Autodesk Inventor part; units mm, degrees
ref_plane "作業平面2" through (-125.5285, -9.35, -169.7679) normal (-0.3826834, 0, 0.9238795) x (0.9238795, 0, 0.3826834)
ref_plane "作業平面4" through (-114.2638, -8.3771, -110.4647) normal (0, 0, 1) x (1, 0, 0)
ref_plane "YZ Plane" through (0, 0, 0) normal (1, 0, 0) x (0, 1, 0)
ref_plane "作業平面1" through (-58.5419, 13.75, 0) normal (0, 0, -1) x (-1, 0, 0)
sketch "スケッチ1" plane through (-58.5419, 13.75, 0) normal (0, 0, -1) x (-1, 0, 0)
  line L0 (-47.5988, 17.4243) -> (46.6818, -19.75)
  line L1 (46.6818, -19.75) -> (47.5988, -17.4243)
  line L2 (47.5988, -17.4243) -> (-46.6818, 19.75)
  line L3 (-46.6818, 19.75) -> (-47.5988, 17.4243)
  point P0 (-58.5419, -13.75)
ref_plane "作業平面2" through (-125.5285, -9.35, -169.7679) normal (-0.3826834, 0, 0.9238795) x (0.9238795, 0, 0.3826834)
extrude "押し出し1" add sketch "スケッチ1" along normal up to surface surface through (-125.5285, -9.35, -169.7679) normal (-0.3826834, 0, 0.9238795)
sketch "スケッチ2" plane through (-106.1408, -3.6743, 0) normal (-0.3668097, 0.930296, 0) x (0.930296, 0.3668097, 0)
  circle A0 centre (76.1355, 115.4647) radius 1.5
  circle A1 centre (45.616, 115.4647) radius 1.5
  line L0 (30.3562, 120.4647) -> (30.3562, 110.4647)
  line L1 (91.3953, 120.4647) -> (30.3562, 120.4647)
  line L2 (91.3953, 110.4647) -> (91.3953, 120.4647)
  line L3 (30.3562, 110.4647) -> (91.3953, 110.4647)
  circle A2 centre (76.1355, 5) radius 1.5
  circle A3 centre (45.616, 5) radius 1.5
  line L4 (30.3562, 10) -> (30.3562, 0)
  line L5 (91.3953, 10) -> (30.3562, 10)
  line L6 (91.3953, 0) -> (91.3953, 10)
  line L7 (30.3562, 0) -> (91.3953, 0)
  point P0 (100.0901, 0)
extrude "押し出し2" cut sketch "スケッチ2" against normal blind 10 contours A0 | A1 | A2 | A3
ref_plane "作業平面3" through (-60.4061, 12.6229, -10) normal (0, 0, -1) x (-1, 0, 0)
sketch "スケッチ3" plane through (-60.4061, 12.6229, -10) normal (0, 0, -1) x (-1, 0, 0)
  line L0 (53.8577, -19.5) -> (45.423, -16.1743)
  line L1 (53.8577, -21) -> (53.8577, -19.5)
  line L2 (-53.8577, -21) -> (53.8577, -21)
  line L3 (44.8176, -18.6229) -> (45.7346, -16.2971)
  line L4 (45.7346, -16.2971) -> (44.8176, -18.6229)
  line L5 (44.8176, -18.6229) -> (50.8464, -21)
  line L6 (50.8464, -21) -> (51.7634, -18.6743)
  line L7 (51.7634, -18.6743) -> (45.7346, -16.2971)
  point P0 (-60.4061, -12.6229)
  point P1 (44.506, -18.5)
  point P2 (51.7634, -18.6743)
ref_plane "作業平面4" through (-114.2638, -8.3771, -110.4647) normal (0, 0, 1) x (1, 0, 0)
extrude "押し出し3" add sketch "スケッチ3" along normal up to surface (100.4647 mm away) contours L6 L5 L3 L0
ref_plane "作業平面5" through (-60.4061, 12.6229, -120.4647) normal (0, 0, -1) x (-1, 0, 0)
sketch "スケッチ4" plane through (-60.4061, 12.6229, -120.4647) normal (0, 0, -1) x (-1, 0, 0)
  line L0 (50.8464, -21) -> (51.7634, -18.6743)
  line L1 (44.8176, -18.6229) -> (45.7346, -16.2971)
  line L2 (53.8577, -19.5) -> (45.423, -16.1743)
  line L3 (44.8176, -18.6229) -> (50.8464, -21)
  point P0 (-60.4061, -12.6229)
extrude "押し出し4" add sketch "スケッチ4" along normal up to surface surface through (-58.5419, 13.75, -142.0212) normal (-0.3826834, 0, 0.9238795)
sketch "スケッチ6" plane through (-11.8601, 33.5, 0) normal (-0.3668097, 0.930296, 0) x (0.930296, 0.3668097, 0)
  line L0 (-107.8253, 164.2345) -> (0, 122.685)
  line L1 (0, 0) -> (0, 122.685)
  line L2 (-107.8253, 120.4647) -> (-107.8253, 164.2345)
  line L3 (-107.8253, 163.6987) -> (0, 122.1491)
  point P0 (-1.2547, 0)
  dimension "d9" = 0.5
extrude "押し出し5" cut sketch "スケッチ6" against normal blind 2.5
properties part number "Right_Wall" material "木材 (カエデ材)"
Geometry: final body of the model. Coordinates: model frame, mm. Round coordinates to 2 decimals unless told otherwise and drop trailing zeros. Loops run counter-clockwise (first coordinate to the right, second up) from the corner with the lowest first, then second, coordinate; pieces in that order, holes last.
Q1. Section A-A on z = -89.5. Return loops of the section in (x, y), plus the area to 3 significant figures.
Q2. Pin query (flat end, axial travel): P1, Ø3, axis at x = -62, y = 11, coming from the -Z side; P2, Ø1.4, axis at x = -108.5, y = -7, coming from the +Z side; P3, Ø12, axis at y = -3.5, z = -27.5, coming from the -X side. Return the tip coordinate at first contact, or that it passes through.
Q3. Section B-B on y = 3. Return loops of the section in (x, z).
Q4. Section C-C on x = -23. Return loops of the section in (y, z), plus the area to 3 significant figures.
Q5. Section D-D on z = -139.5. Return loops of the section in (x, y).
Q6. Pull-direction query (Z, two-part tool) for faces 1 (the flat face through (-109, -6, -120.465)), 2 (the flat face through (-62.265, 12.301, -143.215)), 3 (the flat face through (-58, 14, 0)); classes: released by +Z, released by -Z, zero draft, split by the parting line, or undercut.
Q7. Material intervals for L1, parallel to Y at x = -68.5, z = -24; L2, parallel to Y at x = -65, z = -44, sorted ascending.
Evaluation:
1. outline: (-112.17, -6.05) - (-111.25, -8.38) - (-105.22, -6) - (-10.94, 31.17) - (-11.86, 33.5) - (-106.14, -3.67) - close
1. area: 270 mm2
2. P1: stops at z = -143.88
2. P2: stops at z = -10
2. P3: stops at x = -112.17
3. outline: (-89.21, -154.19) - (-82.4, -151.75) - (-82.4, 0) - (-89.21, 0) - close
4. outline: (26.42, -127.14) - (29.11, -126.76) - (29.11, 0) - (26.42, 0) - close
4. area: 341 mm2
5. outline: (-112.17, -6.05) - (-111.25, -8.38) - (-105.22, -6) - (-52.83, 14.66) - (-53.75, 16.98) - (-106.14, -3.67) - close
6. face 1: undercut
6. face 2: released by -Z
6. face 3: released by +Z
7. L1: y = 8.48 to 11.17
7. L2: y = 9.86 to 12.55
